```python
from build123d import *

# Parameters (mm, degrees)
SKETCH1_W                = 127
SKETCH1_H                = 127
BOSS_EXTRUDE1_DEPTH      = 2.4
SKETCH2_W                = 26.4
SKETCH2_H                = 15
BOSS_EXTRUDE3_DEPTH      = 5.5
BOSS_EXTRUDE4_REACH      = 92.149
BOSS_EXTRUDE4_END_RADIUS = 8
SKETCH3_W                = 26.4
SKETCH3_H                = 12.8
SKETCH4_W                = 26.4
SKETCH4_H                = 1.1
BOSS_EXTRUDE5_DEPTH      = 13.40885
BOSS_EXTRUDE8_DEPTH      = 7
SKETCH7_R                = 0.8
BOSS_EXTRUDE9_DEPTH      = 3
SKETCH8_R                = 1.25
BOSS_EXTRUDE10_DEPTH     = 3
SKETCH9_W                = 5.6
SKETCH9_H                = 10
BOSS_EXTRUDE11_DEPTH     = 21
SKETCH10_R               = 1.7
CUT_EXTRUDE1_DEPTH       = 5.6
BOSS_EXTRUDE12_DEPTH     = 127


with BuildPart() as part:
    # Sketch1 → Boss-Extrude1 (new body)
    with BuildSketch(Plane(origin=(0, 0, 0), x_dir=(1, 0, 0), z_dir=(0, 1, 0))):
        Rectangle(SKETCH1_W, SKETCH1_H)
    extrude(amount=BOSS_EXTRUDE1_DEPTH)

    # Sketch2 → Boss-Extrude3 (add)
    with BuildSketch(Plane(origin=(0, 2.4, 0), x_dir=(1, 0, 0), z_dir=(0, 1, 0))):
        with Locations((-39.747989038, -50.434775134)):
            Rectangle(SKETCH2_W, SKETCH2_H)
    boss_extrude3 = extrude(amount=BOSS_EXTRUDE3_DEPTH)

    # Boss-Extrude4: up to this cylinder (the profile starts outside it)
    boss_extrude4_end = Plane(origin=(-39.747989, 15.906072529, 50.434775134), z_dir=(-1, 0, 0)) * Cylinder(BOSS_EXTRUDE4_END_RADIUS, 201.298, mode=Mode.PRIVATE)
    # Sketch3 → Boss-Extrude4 (add, up to the surface)
    with BuildSketch(Plane(origin=(0, 7.9, 0), x_dir=(1, 0, 0), z_dir=(0, 1, 0)), mode=Mode.PRIVATE) as boss_extrude4_sk1:
        with Locations((-39.747989038, -50.434775134)):
            Rectangle(SKETCH3_W, SKETCH3_H)
    boss_extrude4_tool1 = extrude(boss_extrude4_sk1.sketch, amount=BOSS_EXTRUDE4_REACH, mode=Mode.PRIVATE) - boss_extrude4_end
    boss_extrude4 = boss_extrude4_tool1.solids().sort_by_distance((-39.747989, 7.9, 50.434775))[0]
    add(boss_extrude4)

    # Sketch4 → Boss-Extrude5 (add)
    with BuildSketch(Plane(origin=(0, 7.9, 0), x_dir=(1, 0, 0), z_dir=(0, 1, 0))):
        with Locations((-39.747989038, -43.484775134)):
            Rectangle(SKETCH4_W, SKETCH4_H)
        with Locations((-39.747989038, -57.384775134)):
            Rectangle(SKETCH4_W, SKETCH4_H)
    boss_extrude5 = extrude(amount=BOSS_EXTRUDE5_DEPTH)

    # Mirror1: Boss-Extrude3 across plane
    add(boss_extrude3.mirror(Plane(origin=(0, 0, 0), x_dir=(0, 0, 1), z_dir=(1, 0, 0))))

    # Mirror2: Boss-Extrude5 across plane
    add(boss_extrude5.mirror(Plane(origin=(0, 0, 0), x_dir=(0, 0, 1), z_dir=(1, 0, 0))))

    # Mirror3: Boss-Extrude4 across plane
    add(boss_extrude4.mirror(Plane(origin=(0, 0, 0), x_dir=(0, 0, 1), z_dir=(1, 0, 0))))

    # Sketch6 → Boss-Extrude8 (add)
    with BuildSketch(Plane(origin=(0, 2.4, 0), x_dir=(1, 0, 0), z_dir=(0, 1, 0))):
        Polygon((-58.25637406, -39.71881472), (-58.25637406, -40.71881472), (-38.943651891, -40.71881472), (-38.943651891, 22.696046836), (-39.943651891, 22.696046836), (-39.943651891, -39.71881472), align=None)
    extrude(amount=BOSS_EXTRUDE8_DEPTH)

    # Sketch7 → Boss-Extrude9 (add)
    with BuildSketch(Plane(origin=(0, 2.4, 0), x_dir=(1, 0, 0), z_dir=(0, 1, 0))):
        with Locations(Location((-20.157758856, -36.323995409, 0), (0, 0, 90))):
            Circle(SKETCH7_R)
        with Locations(Location((-35.457758856, -36.323995409, 0), (0, 0, 90))):
            Circle(SKETCH7_R)
        with Locations(Location((-14.70070569, -60.698401589, 0), (0, 0, 90))):
            Circle(SKETCH7_R)
        with Locations(Location((0.59929431, -60.698401589, 0), (0, 0, 90))):
            Circle(SKETCH7_R)
    extrude(amount=BOSS_EXTRUDE9_DEPTH)

    # Sketch8 → Boss-Extrude10 (add)
    with BuildSketch(Plane(origin=(0, 2.4, 0), x_dir=(1, 0, 0), z_dir=(0, 1, 0))):
        with Locations(Location((-10.411058541, -6.196769083, 0), (0, 0, 90))):
            Circle(SKETCH8_R)
    extrude(amount=BOSS_EXTRUDE10_DEPTH)

    # Sketch9 → Boss-Extrude11 (add)
    with BuildSketch(Plane(origin=(0, 2.4, 0), x_dir=(1, 0, 0), z_dir=(0, 1, 0))):
        with Locations((21.5, 3.5)):
            Rectangle(SKETCH9_W, SKETCH9_H)
    extrude(amount=BOSS_EXTRUDE11_DEPTH)

    # Sketch10 → Cut-Extrude1 (cut)
    with BuildSketch(Plane(origin=(24.3, 0, 0), x_dir=(0, 0, -1), z_dir=(1, 0, 0))):
        with Locations((3.3, 17.35)):
            Circle(SKETCH10_R)
        with Locations((3.3, 7.45)):
            Circle(SKETCH10_R)
    extrude(amount=-CUT_EXTRUDE1_DEPTH, mode=Mode.SUBTRACT)

    # Sketch11 → Boss-Extrude12 (add)
    with BuildSketch(Plane(origin=(63.5, 0, 0), x_dir=(0, 0, -1), z_dir=(1, 0, 0))):
        Polygon((63.5, 2.4), (67.656921938, 0), (63.5, 0), align=None)
    extrude(amount=-BOSS_EXTRUDE12_DEPTH)


solid = part.part
```
Model file for the job. Use its own axes, mm. A direction names the side the tool comes from. Give positions to 0.01 mm unless a question says otherwise; leave off trailing zeros. Write each loop counter-clockwise with the first axis right and the second up, starting at its lowest first coordinate (ties: lowest second). Pieces come first, ordered by that corner, then holes. Notation, with made-up numbers: (15.25, 62.5) -> (24.25, 62.5) arc R25 ccw to (24.25, 88.5) -> close; hole circle Ø3 at (38, 83.5). An arc over 180 degrees is marked (long way). Use CSV: the item, a comma, the result in double quotes. Start each with the question number.
1) Pin check, flat tips, straight feed: P1, Ø0.5, axis at x = -36, z = 36.5, coming from the +Y side; P2, Ø6, axis at x = 20.5, y = 8.5, coming from the +Z side; P3, Ø3, axis at x = 40.5, y = 16, coming from the -Z side; P4, Ø3, axis at y = 3.5, z = 29.5, coming from the -X side. Stop position of each tip, or through.
2) Tool access for faces 4 (the flat face through (40, 12, 42.935)), 5 (the flat face through (-39.3, 9.4, 8.9)), 6 (the cylindrical face through (21.539, 9.136, -3.079)): list every direction of +Z, -Z, +X, -X, +Y, -Y with a clear straight run to the whole face (end or side of a thin tool).
3) Cut at D-D on x = 14.5. List the corners of the cut face in (y, z).
4) Two-plate mould, pull along Z, no slides. Class faces 1 (the flat face through (40, 16, 44.035)), 2 (the flat face through (1, 0, -3)), 3 (the flat face through (21, 13, 1.5)): released by +Z, released by -Z, zero draft, split by the parting line, or undercut.
5) Cut at B-B on z = -3.3. List the corners of the cut face in (x, y).
6) Drill centre lines: L1, parallel to X at y = 8, z = 57; L2, parallel to Z at x = -52.5, y = 12.5; L3, parallel to X at y = 7.25, z = -9. Where is each one in solid material? Low to high.
7) Cut at A-A on y = 17.35. List the corners of the cut face in (x, z), plus the area to 3 significant figures.
8) Cut at C-C on z = 50.5. List the corners of the cut face in (x, y), plus the area to 3 significant figures.
Final values:
1,P1,"stops at y = 5.4"
1,P2,"stops at z = 1.5"
1,P3,"stops at z = 42.93"
1,P4,"stops at x = -63.5"
2,face 4,"-Z, +X, -X, +Y"
2,face 5,"-Z, -X, +Y"
2,face 6,"+X"
3,outline,"(0, -67.66) -> (2.4, -63.5) -> (2.4, 63.5) -> (0, 63.5) -> close"
4,face 1,"undercut"
4,face 2,"zero draft"
4,face 3,"released by +Z"
5,outline,"(-63.5, 0) -> (63.5, 0) -> (63.5, 2.4) -> (24.3, 2.4) -> (24.3, 5.75) -> (18.7, 5.75) -> (18.7, 2.4) -> (-38.94, 2.4) -> (-38.94, 9.4) -> (-39.94, 9.4) -> (-39.94, 2.4) -> (-63.5, 2.4) -> close; (18.7, 9.15) -> (24.3, 9.15) -> (24.3, 15.65) -> (18.7, 15.65) -> close; (18.7, 19.05) -> (24.3, 19.05) -> (24.3, 23.4) -> (18.7, 23.4) -> close"
6,L1,"x = -52.95 to -26.55, 26.55 to 52.95"
6,L2,"z = 42.93 to 44.03, 56.83 to 57.93"
6,L3,"x = -39.94 to -38.94"
7,outline,"(-52.95, 42.93) -> (-26.55, 42.93) -> (-26.55, 44.03) -> (-52.95, 44.03) -> close; (-52.95, 56.83) -> (-26.55, 56.83) -> (-26.55, 57.93) -> (-52.95, 57.93) -> close; (18.7, -8.5) -> (24.3, -8.5) -> (24.3, -5) -> (18.7, -5) -> close; (18.7, -1.6) -> (24.3, -1.6) -> (24.3, 1.5) -> (18.7, 1.5) -> close; (26.55, 42.93) -> (52.95, 42.93) -> (52.95, 44.03) -> (26.55, 44.03) -> close; (26.55, 56.83) -> (52.95, 56.83) -> (52.95, 57.93) -> (26.55, 57.93) -> close"
7,area,"153 mm2"
8,outline,"(-63.5, 0) -> (63.5, 0) -> (63.5, 2.4) -> (52.95, 2.4) -> (52.95, 7.91) -> (26.55, 7.91) -> (26.55, 2.4) -> (-26.55, 2.4) -> (-26.55, 7.91) -> (-52.95, 7.91) -> (-52.95, 2.4) -> (-63.5, 2.4) -> close"
8,area,"596 mm2"
